from build123d import *

# Parameters (mm, degrees)
SKETCH1_R                            = 4.7625
BOSS_EXTRUDE1_DEPTH                  = 304.8
F_10_32_TAPPED_HOLE1_D               = 4.0386
F_10_32_TAPPED_HOLE1_DEPTH           = 12.02944
F_10_32_TAPPED_HOLE1_TIP             = 1.213317848
F_10_32_TAPPED_HOLE1_ON_FACE_2_D     = 4.0386
F_10_32_TAPPED_HOLE1_ON_FACE_2_DEPTH = 12.02944
F_10_32_TAPPED_HOLE1_ON_FACE_2_TIP   = 1.213317848


with BuildPart() as part:
    # Sketch1 → Boss-Extrude1 (new, symmetric)
    with BuildSketch(Plane.XY):
        with Locations(Location((0, 0, 0), (0, 0, 180))):
            Circle(SKETCH1_R)
    extrude(amount=BOSS_EXTRUDE1_DEPTH, both=True)

    # #10-32 Tapped Hole1
    with Locations(Plane(origin=(0, 0, -304.8), x_dir=(-1, 0, 0), z_dir=(0, 0, -1))):
        with Locations((0, 0)):
            Hole(F_10_32_TAPPED_HOLE1_D / 2, depth=F_10_32_TAPPED_HOLE1_DEPTH)
            with Locations((0, 0, -(F_10_32_TAPPED_HOLE1_DEPTH + F_10_32_TAPPED_HOLE1_TIP / 2))):  # 118° drill point
                Cone(0, F_10_32_TAPPED_HOLE1_D / 2, F_10_32_TAPPED_HOLE1_TIP, mode=Mode.SUBTRACT)

    # #10-32 Tapped Hole1 on face 2
    with Locations(Plane.XY.offset(304.8)):
        with Locations((0, 0)):
            Hole(F_10_32_TAPPED_HOLE1_ON_FACE_2_D / 2, depth=F_10_32_TAPPED_HOLE1_ON_FACE_2_DEPTH)
            with Locations((0, 0, -(F_10_32_TAPPED_HOLE1_ON_FACE_2_DEPTH + F_10_32_TAPPED_HOLE1_ON_FACE_2_TIP / 2))):  # 118° drill point
                Cone(0, F_10_32_TAPPED_HOLE1_ON_FACE_2_D / 2, F_10_32_TAPPED_HOLE1_ON_FACE_2_TIP, mode=Mode.SUBTRACT)


solid = part.part
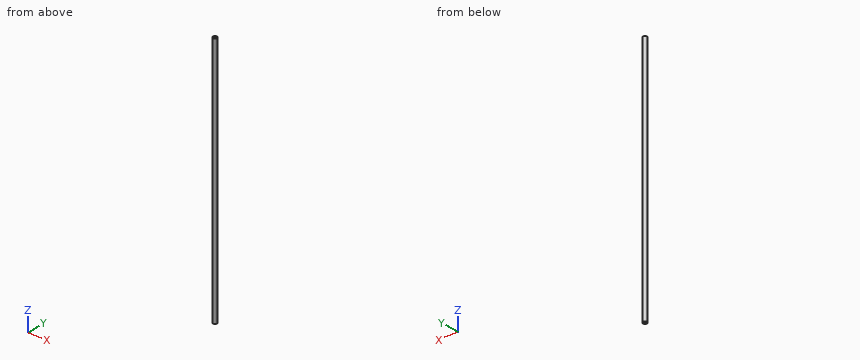
Input: part model. Units: mm. Frame: model coordinates. Round coordinates to 2 decimals unless told otherwise and drop trailing zeros. Write each loop counter-clockwise with the first axis right and the second up, starting at its lowest first coordinate (ties: lowest second). Pieces come first, ordered by that corner, then holes.
1) Ray query, L1, parallel to Y at x = 0, z = -295.25; L2, parallel to Y at x = -0.25, z = 271.5; L3, parallel to X at y = 0.75, z = -123. Return the intervals inside material, ascending.
2) Cut plane A-A (z = 6). Return the cut outline in (x, y) (1 decimal), then the cut area to 3 significant figures.
3) Contact query for flat-ended pins moving along their axis: P1, Ø3, axis at x = 1.5, y = -1, coming from the -Z side; P2, Ø5, axis at x = 3, z = 35.5, coming from the -Y side; P3, Ø1.5, axis at x = 2.5, z = 2.5, coming from the -Y side; P4, Ø2.5, axis at x = 0, y = 0, coming from the -Z side. Output: stop coordinate, or through.
Geometry says:
1. L1: y = -4.76 to -2.02, 2.02 to 4.76
1. L2: y = -4.76 to 4.76
1. L3: x = -4.7 to 4.7
2. outline: circle Ø9.5 at (0, 0)
2. area: 71.3 mm2
3. P1: stops at z = -304.8
3. P2: stops at y = -4.74
3. P3: stops at y = -4.43
3. P4: stops at z = -292.31
